Verification items for the finished model (mm, model axes). Face numbers are marked on the shaded views. A direction names the side the tool comes from. Round coordinates to 2 decimals unless told otherwise and drop trailing zeros. Loops run counter-clockwise (first coordinate to the right, second up) from the corner with the lowest first, then second, coordinate; pieces in that order, holes last. Notation, with made-up numbers: (-9.5, -24.5) - (42.5, -24.5) arc R26 cw to (42.5, -8.5) - close; hole circle Ø1 at (7.25, 6). An arc over 180 degrees is marked (long way). Use CSV: the item, a comma, the result in double quotes.
```python
from build123d import *

# Parameters (mm, degrees)
F1_DEPTH = 20
F2_R     = 1
F3_R     = 1


with BuildPart() as f1:
    # F0 (on Front) → F1 (new body)
    with BuildSketch(Plane.XZ):
        Polygon((10, 13), (10, 16), (0, 16), (0, 0), (10, 0), (10, 3), (2, 2), (2, 14), align=None)
    extrude(amount=F1_DEPTH)

    # F2
    f2_edges = [f1.edges().sort_by_distance(p)[0] for p in [
        (10, -10, 13),
        (10, -10, 3),
        (2, -10, 14),
        (2, -10, 2),
    ]]
    fillet(f2_edges, radius=F2_R)

    # F3
    f3_edges = [f1.edges().sort_by_distance(p)[0] for p in [
        (0, -10, 0),
        (0, -10, 16),
    ]]
    fillet(f3_edges, radius=F3_R)


solid = f1.part
```
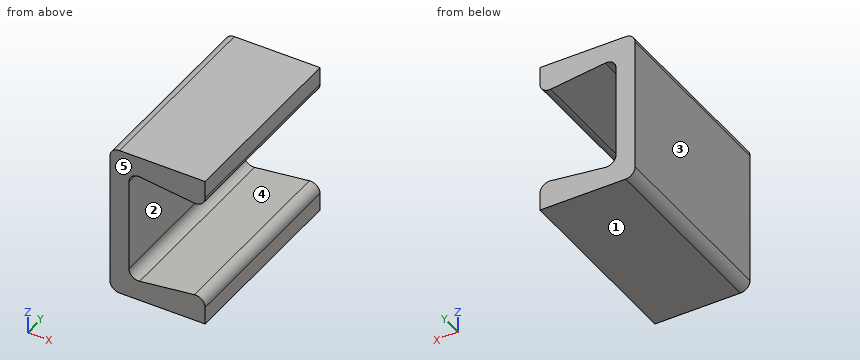
1) Cross-section at B-B, the plane y = -11.5. Record the cut outline in (x, z), then the cut area to 3 significant figures.
Returned:
outline,"(0, 1) arc R1 ccw to (1, 0) - (10, 0) - (10, 1.87) arc R1 ccw to (8.88, 2.86) - (3.12, 2.14) arc R1 cw to (2, 3.13) - (2, 12.87) arc R1 cw to (3.12, 13.86) - (8.88, 13.14) arc R1 ccw to (10, 14.13) - (10, 16) - (1, 16) arc R1 ccw to (0, 15) - close"
area,"71.6 mm²"
2) Mould release check, pull along Z, two halves, no side actions. Record for the marked faces 1, 2 and 3: +Z half, -Z half, draft (parallel to the pull), parting line (faces both ways), or undercut.
Returned:
face 1,"-Z half"
face 2,"undercut"
face 3,"draft"
3) Cross-section at C-C, the plane z = 13.5. Record the cut outline in (x, y).
Returned:
outline,"(0, -20) - (2.23, -20) - (2.23, 0) - (0, 0) - close; (6, -20) - (9.77, -20) - (9.77, 0) - (6, 0) - close"
4) Access from +Z, -Z, +X, -X, +Y, -Y to the whole of each face (thin tool, end or side, straight path). Record for the marked faces 4 and 5.
Returned:
face 4,"+Y, -Y"
face 5,"+Z, -Z, +X, -X, -Y"
5) Thickness scan on probe 1 along Z at (x, y) = (3, -16); probe 2 along X at (y, z) = (-14, 3.25); probe 3 along Z at (x, y) = (7.25, -17). Record the ranges inside material, lowest first. Write a range as [from, to].
Returned:
probe 1,"z = [0, 2.13], [13.87, 16]"
probe 2,"x = [0, 2]"
probe 3,"z = [0, 2.66], [13.34, 16]"
6) Cross-section at A-A, the plane x = 7.5. Record the cut outline in (y, z), then the cut area to 4 significant figures.
Returned:
outline,"(-20, 0) - (0, 0) - (0, 2.69) - (-20, 2.69) - close; (-20, 13.31) - (0, 13.31) - (0, 16) - (-20, 16) - close"
area,"107.5 mm²"
7) Gauge pin test, flat ends, axial feed: pin 1 Ø5 at (y, z) = (-16.5, 3.5) entering from +X; pin 2 Ø8 at (y, z) = (-10, 9.5) entering from +X; pin 3 Ø1 at (y, z) = (-15.5, 8) entering from +X. Record the tip position at first contact, or that the pin passes through.
Returned:
pin 1,"stops at x = 10"
pin 2,"stops at x = 9.77"
pin 3,"stops at x = 2"
